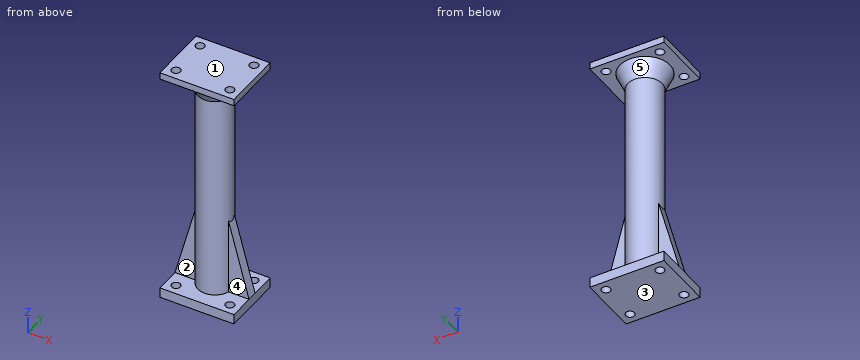
from build123d import *

# Parameters (mm, degrees)
SKETCH1_W           = 22
SKETCH1_H           = 18
SKETCH1_R           = 5.1
SKETCH1_R_2         = 1.3
BOSS_EXTRUDE1_DEPTH = 3
SKETCH1_3_R         = 5.1
BOSS_EXTRUDE2_DEPTH = 70
SKETCH2_W           = 22
SKETCH2_H           = 18
SKETCH2_R           = 1.3
BOSS_EXTRUDE3_DEPTH = 2
CHAMFER2_SIZE       = 5
CHAMFER2_SIZE2      = 2.331538291
RIB2_REACH          = 75.389
SKETCH3_WALL_W      = 171.556146136
SKETCH3_WALL_H      = 3
RIB3_REACH          = 75.389
SKETCH4_WALL_W      = 171.556146136
SKETCH4_WALL_H      = 3


with BuildPart() as part:
    # Sketch1 → Boss-Extrude1 (new body)
    with BuildSketch(Plane.XY):
        Rectangle(SKETCH1_W, SKETCH1_H)
        Circle(SKETCH1_R, mode=Mode.SUBTRACT)
        with Locations((-8, 6)):
            Circle(SKETCH1_R_2, mode=Mode.SUBTRACT)
        with Locations((8, 6)):
            Circle(SKETCH1_R_2, mode=Mode.SUBTRACT)
        with Locations((8, -6)):
            Circle(SKETCH1_R_2, mode=Mode.SUBTRACT)
        with Locations((-8, -6)):
            Circle(SKETCH1_R_2, mode=Mode.SUBTRACT)
    extrude(amount=BOSS_EXTRUDE1_DEPTH)

    # Sketch1_3 → Boss-Extrude2 (add)
    with BuildSketch(Plane.XY):
        Circle(SKETCH1_3_R)
    extrude(amount=BOSS_EXTRUDE2_DEPTH)

    # Sketch2 → Boss-Extrude3 (add)
    with BuildSketch(Plane.XY.offset(70)):
        Rectangle(SKETCH2_W, SKETCH2_H)
        with Locations((-8, 6)):
            Circle(SKETCH2_R, mode=Mode.SUBTRACT)
        with Locations((8, 6)):
            Circle(SKETCH2_R, mode=Mode.SUBTRACT)
        with Locations((8, -6)):
            Circle(SKETCH2_R, mode=Mode.SUBTRACT)
        with Locations((-8, -6)):
            Circle(SKETCH2_R, mode=Mode.SUBTRACT)
    extrude(amount=BOSS_EXTRUDE3_DEPTH)

    # Chamfer2
    chamfer2_edges = [part.edges().sort_by_distance(p)[0] for p in [
        (-5.1, 0, 70),
    ]]
    chamfer2_side = [part.faces().sort_by_distance(p)[0] for p in [
        (-5.1, 0, 36.5),
    ]]
    chamfer(chamfer2_edges, length=CHAMFER2_SIZE, length2=CHAMFER2_SIZE2, reference=chamfer2_side[0])

    # Sketch3 wall → Rib2 (add, up to next)
    with BuildSketch(Plane(origin=(-8.05, 0, 14), x_dir=(0.259028674037, 0, 0.965869632003), z_dir=(0.965869632003, 0, -0.259028674037)), mode=Mode.PRIVATE) as rib2_sk1:
        Rectangle(SKETCH3_WALL_W, SKETCH3_WALL_H)
    rib2_tool1 = extrude(rib2_sk1.sketch, amount=RIB2_REACH, mode=Mode.PRIVATE) - part.part
    add(rib2_tool1.solids().sort_by_distance((-8.05, 0, 14))[0])

    # Sketch4 wall → Rib3 (add, up to next)
    with BuildSketch(Plane(origin=(8.05, 0, 14), x_dir=(-0.259028674037, 0, 0.965869632003), z_dir=(0.965869632003, 0, 0.259028674037)), mode=Mode.PRIVATE) as rib3_sk1:
        Rectangle(SKETCH4_WALL_W, SKETCH4_WALL_H)
    rib3_tool1 = extrude(rib3_sk1.sketch, amount=-RIB3_REACH, mode=Mode.PRIVATE) - part.part
    add(rib3_tool1.solids().sort_by_distance((8.05, 0, 14))[0])


solid = part.part
Verification items for the finished model (mm, model axes). Face numbers are marked on the shaded views. A direction names the side the tool comes from. Coordinates: 2 decimals unless noted, no trailing zeros. Loops run counter-clockwise (first coordinate to the right, second up) from the corner with the lowest first, then second, coordinate; pieces in that order, holes last. Notation, with made-up numbers: M 61,29.5 L 93,29.5 A14 cw 93,54.5 Z; hole C -5,-10.75 d5. An arc over 180 degrees is marked long. One line per item, written item: value.
1. Set-up check for the marked faces 4 and 5: record each of +Z, -Z, +X, -X, +Y, -Y from which the full face is reachable in a straight line by a thin tool's end or side.
Answers follow:
face 4: +X, -Y
face 5: none
2. Section check C-C on z = 34. Record the cut outline in (x, y).
Answers follow:
outline: C 0,0 d10.2
3. Gauge pin test, flat ends, axial feed: P1, Ø5, axis at x = 8.5, z = 16, coming from the -Y side; P2, Ø5, axis at x = -7.5, z = 19, coming from the +Y side; P3, Ø4, axis at x = 3, z = 56, coming from the +Y side. Record the tip position at first contact, or that the pin passes through.
Answers follow:
P1: y = -1.5
P2: y = 1.5
P3: y = 5
4. Section check D-D on y = -6. Give the number of separate pieces and of enclosed holes in the cut face, plus the area to 3 significant figures.
Answers follow:
separate pieces: 6
enclosed holes: 0
area: 102 mm^2
5. Section check A-A on y = 0. Record the cut outline in (x, z), plus the area to 3 significant figures.
Answers follow:
outline: M -11,0 L 11,0 L 11,3 L 5.1,25 L 5.1,65 L 7.43,70 L 11,70 L 11,72 L -11,72 L -11,70 L -7.43,70 L -5.1,65 L -5.1,25 L -11,3 Z
area: 935 mm^2
6. Material ranges on line 1 along Y through (x, z) = (8, 1.6); line 2 along Z through (x, y) = (5, -5.5); line 3 along Y through (x, z) = (5.5, 4), recorded low to high. Write a range as from..to.
Answers follow:
line 1: -9..-7.3, -4.7..4.7, 7.3..9
line 2: 0..3, 70..72
line 3: -1.5..1.5
7. Section check B-B on x = 0. Record the cut outline in (y, z).
Answers follow:
outline: M -9,0 L 9,0 L 9,3 L 5.1,3 L 5.1,65 L 7.43,70 L 9,70 L 9,72 L -9,72 L -9,70 L -7.43,70 L -5.1,65 L -5.1,3 L -9,3 Z
8. Mould release check, pull along Z, two halves, no side actions. Record for the marked faces 1, 2 and 3: pulls with the +Z half, pulls with the -Z half, needs draft (parallel to the pull), parting line crosses it, or undercut.
Answers follow:
face 1: pulls with the +Z half
face 2: undercut
face 3: pulls with the -Z half
